Answer from the drawing. Dimensions are ordinates in mm from the lowest x, y and z of the part. Coordinates: 2 decimals unless noted, no trailing zeros. Write each loop counter-clockwise with the first axis right and the second up, starting at its lowest first coordinate (ties: lowest second). Pieces come first, ordered by that corner, then holes. Notation, with made-up numbers: (45, 61) - (101, 61) arc R12 ccw to (101, 83) - close; hole circle Ø6 at (68.25, 41.25). An arc over 180 degrees is marked (long way). Answer as a JSON object with one key per item and string values. Group by question number.
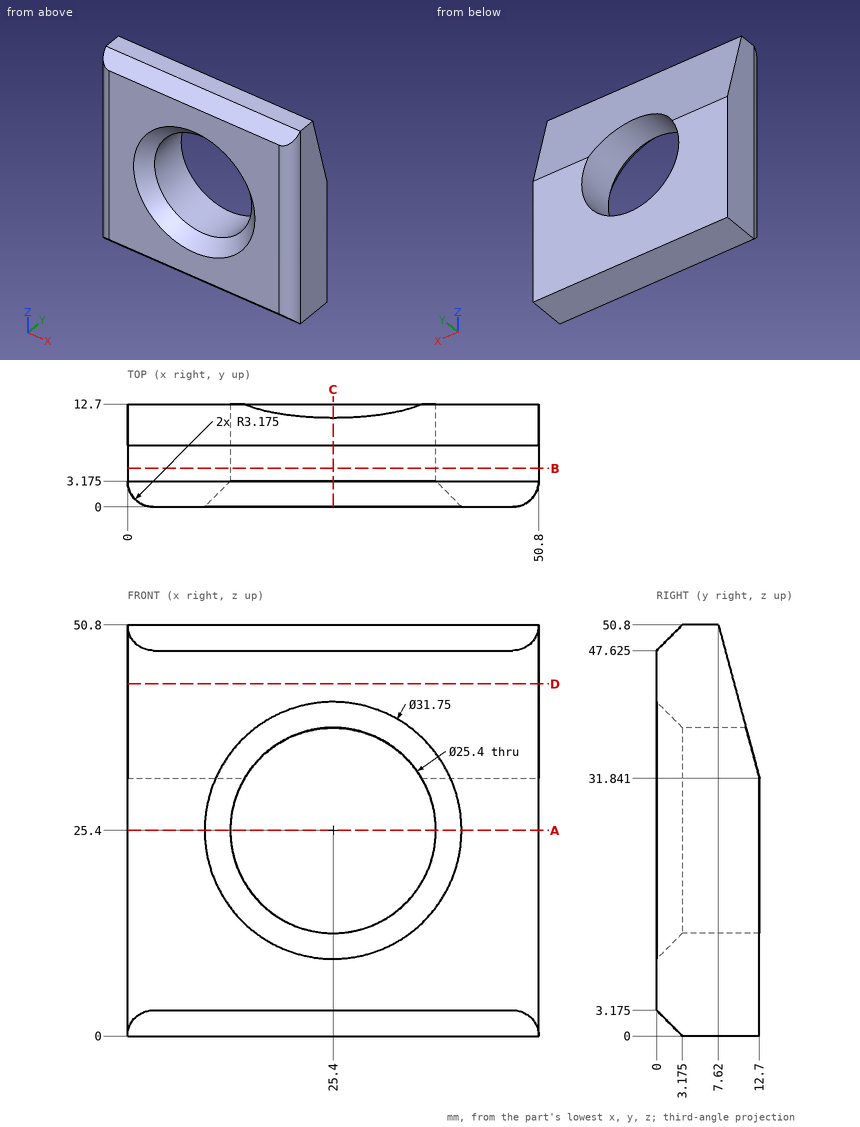
Q1. Section B-B on y = 4.75 is taken. Determine the outline of the cut face in (x, z).
Q2. Section D-D on z = 43.5 is taken. Determine the outline of the cut face in (x, y) (3 decimals), plus the area to 3 significant figures.
Q3. Consider L1, parallel to Z at x = 25.4, y = 6; L2, parallel to Z at x = 21.5, y = 7. Determine where each line is inside the solid, lowest interval first. Write a range as from..to.
Q4. Section A-A on z = 25.4 is taken. Determine the outline of the cut face in (x, y) (3 decimals), plus the area to 3 significant figures.
Q5. Section C-C on x = 25.4 is taken. Determine the outline of the cut face in (y, z) (3 decimals), plus the area to 4 significant figures.
Numbers:
{
 "1": {"outline": "(0, 0) - (50.8, 0) - (50.8, 50.8) - (0, 50.8) - close; hole circle Ø25.4 at (25.4, 25.4)"},
 "2": {"outline": "(0, 3.175) arc R3.175 ccw to (3.175, 0) - (47.625, 0) arc R3.175 ccw to (50.8, 3.175) - (50.8, 9.576) - (0, 9.576) - close", "area": "482 mm²"},
 "3": {"L1": "z = 0..12.7, 38.1..50.8", "L2": "z = 0..13.31, 37.49..50.8"},
 "4": {"outline": "(0, 3.175) arc R3.175 ccw to (3.175, 0) - (9.525, 0) - (12.7, 3.175) - (12.7, 12.7) - (0, 12.7) - close; (38.1, 3.175) - (41.275, 0) - (47.625, 0) arc R3.175 ccw to (50.8, 3.175) - (50.8, 12.7) - (38.1, 12.7) - close", "area": "308 mm²"},
 "5": {"outline": "(0, 3.175) - (3.175, 0) - (12.7, 0) - (12.7, 12.7) - (3.175, 12.7) - (0, 9.525) - close; (0, 41.275) - (3.175, 38.1) - (11.023, 38.1) - (7.62, 50.8) - (3.175, 50.8) - (0, 47.625) - close", "area": "259.5 mm²"}
}
